Input: part model. Units: mm. Frame: model coordinates. Face numbers are marked on the shaded views. A direction names the side the tool comes from. Coordinates: 2 decimals unless noted, no trailing zeros. Write each loop counter-clockwise with the first axis right and the second up, starting at its lowest first coordinate (ties: lowest second). Pieces come first, ordered by that corner, then holes. Notation, with made-up numbers: M -32,3 L -7,3 A14 cw -7,24 Z; hole C -35,69 d4. An arc over 180 degrees is marked long. Use CSV: the item, a comma, the result in double quotes.
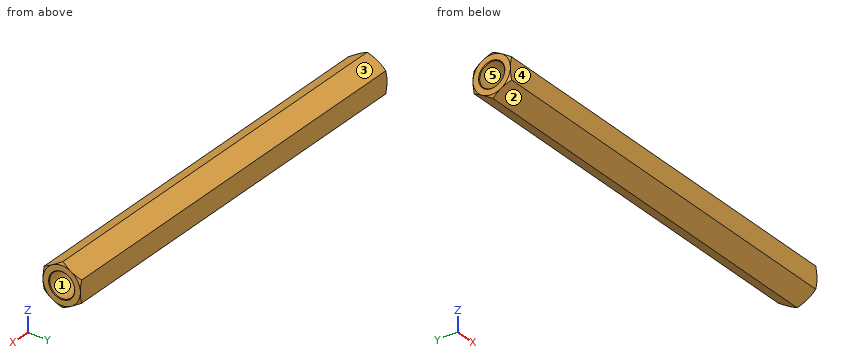
```python
from build123d import *

# Parameters (mm, degrees)
BOSS_EXTRUDE1_DEPTH = 50
SKETCH4_OUTSIDE_W   = 193.96
SKETCH4_OUTSIDE_H   = 193.264
SKETCH4_OUTSIDE_R   = 2.25
CUT_EXTRUDE1_DEPTH  = 51
CUT_EXTRUDE1_TAPER  = 60
SKETCH5_OUTSIDE_W   = 193.96
SKETCH5_OUTSIDE_H   = 193.264
SKETCH5_OUTSIDE_R   = 2.25
CUT_EXTRUDE2_DEPTH  = 51
CUT_EXTRUDE2_TAPER  = 60


with BuildPart() as part:
    # Sketch2 → Boss-Extrude1 (new body)
    with BuildSketch(Plane(origin=(0, 0, 0), x_dir=(0, 0, -1), z_dir=(1, 0, 0))):
        Polygon((1.299038106, 2.25), (-1.299038106, 2.25), (-2.598076211, 0), (-1.299038106, -2.25), (1.299038106, -2.25), (2.598076211, 0), align=None)
    extrude(amount=BOSS_EXTRUDE1_DEPTH)

    # Sketch3 → Cut-Revolve1 (revolve, cut)
    with BuildSketch(Plane.XY):
        Polygon((0, 1.575), (0.075, 1.5), (6.3, 1.5), (6.3, 0), (0, 0), align=None)
        Polygon((50, 0), (43.7, 0), (43.7, 1.5), (49.925, 1.5), (50, 1.575), align=None)
    revolve(axis=Axis((0, 0, 0), (1, 0, 0)), mode=Mode.SUBTRACT)

    # Sketch4 outside → Cut-Extrude1 (cut, through all)
    with BuildSketch(Plane.ZY):
        Rectangle(SKETCH4_OUTSIDE_W, SKETCH4_OUTSIDE_H)
        Circle(SKETCH4_OUTSIDE_R, mode=Mode.SUBTRACT)
    extrude(amount=-CUT_EXTRUDE1_DEPTH, taper=CUT_EXTRUDE1_TAPER, mode=Mode.SUBTRACT)

    # Sketch5 outside → Cut-Extrude2 (cut, through all)
    with BuildSketch(Plane(origin=(50, 0, 0), x_dir=(0, 0, -1), z_dir=(1, 0, 0))):
        Rectangle(SKETCH5_OUTSIDE_W, SKETCH5_OUTSIDE_H)
        Circle(SKETCH5_OUTSIDE_R, mode=Mode.SUBTRACT)
    extrude(amount=-CUT_EXTRUDE2_DEPTH, taper=CUT_EXTRUDE2_TAPER, mode=Mode.SUBTRACT)


solid = part.part
```
1. Mould query, pull axis Y, two halves, no side actions, for the marked faces 3, 4 and 5. Classes: pulls with the +Y half, pulls with the -Y half, needs draft (parallel to the pull), parting line crosses it, or undercut.
Resolved:
face 3,"pulls with the +Y half"
face 4,"pulls with the -Y half"
face 5,"undercut"
2. Access query for the marked faces 1 and 2. Directions: +Z, -Z, +X, -X, +Y, -Y. A direction counts if a zero-diameter tool reaches every point of the face in a straight line with its end or side. Return the directions, or none.
Resolved:
face 1,"+X"
face 2,"-Z, +X, -X, -Y"
3. Section B-B (x = 30). Return loops of the section in (y, z), then the cut area to 3 significant figures.
Resolved:
outline,"M -2.25,-1.3 L 0,-2.6 L 2.25,-1.3 L 2.25,1.3 L 0,2.6 L -2.25,1.3 Z"
area,"17.5 mm^2"
4. Material intervals for line 1 (Z direction, x = 45.75, y = 0); line 2 (Y direction, x = 4.5, z = -0.1); line 3 (X direction, y = 0.9, z = 0.8), sorted ascending. Write a range as [from, to].
Resolved:
line 1,"z = [-2.6, -1.5], [1.5, 2.6]"
line 2,"y = [-2.25, -1.5], [1.5, 2.25]"
line 3,"x = [6.3, 43.7]"
5. Contact query for a flat-ended pin moving along its axis: pin 1 Ø1.5 at (y, z) = (-0.5, 0.5) entering from +X. Output: stop coordinate, or through.
Resolved:
pin 1,"stops at x = 43.7"
6. Section A-A (x = 45.5). Return loops of the section in (y, z), then the cut area to 3 significant figures.
Resolved:
outline,"M -2.25,-1.3 L 0,-2.6 L 2.25,-1.3 L 2.25,1.3 L 0,2.6 L -2.25,1.3 Z; hole C 0,0 d3"
area,"10.5 mm^2"
